The listing builds one solid part. Answer for the finished solid, in the listing's coordinates (mm). A direction names the side the tool comes from. Coordinates: 2 decimals unless noted, no trailing zeros. Loops run counter-clockwise (first coordinate to the right, second up) from the corner with the lowest first, then second, coordinate; pieces in that order, holes last. Notation, with made-up numbers: (-20.5, 42.5) -> (9.5, 42.5) arc R29 cw to (9.5, 80.5) -> close; hole circle Ø7 at (64.5, 76). An arc over 180 degrees is marked (long way). Answer in a Markdown table with one row per item.
```python
from build123d import *

# Parameters (mm, degrees)
F0_W     = 280
F0_H     = 180
F0_R     = 3.25
F0_R_2   = 2.5
F0_R_3   = 5
F0_R_4   = 26
F0_R_5   = 14
F1_DEPTH = 36
F2_DEPTH = 18
F3_DEPTH = 10
F4_D     = 5
F4_DEPTH = 10
F4_TIP   = 1.5021515476
F5_R     = 19
F5_R_2   = 14
F6_DEPTH = 12
F8_R     = 20
F9_DEPTH = 2


with BuildPart() as f1:
    # F0 (on Top) → F1 (new body)
    with BuildSketch(Plane.XY):
        Rectangle(F0_W, F0_H)
        with Locations((-125, -70)):
            Circle(F0_R, mode=Mode.SUBTRACT)
        with Locations((-71.2132034356, -21.2132034356)):
            Circle(F0_R_2, mode=Mode.SUBTRACT)
        with Locations((-28.7867965644, -21.2132034356)):
            Circle(F0_R_2, mode=Mode.SUBTRACT)
        with Locations((125, -70)):
            Circle(F0_R, mode=Mode.SUBTRACT)
        with Locations((125, -55)):
            Circle(F0_R_3, mode=Mode.SUBTRACT)
        with Locations((28.7867965644, -21.2132034356)):
            Circle(F0_R_2, mode=Mode.SUBTRACT)
        with Locations((71.2132034356, -21.2132034356)):
            Circle(F0_R_2, mode=Mode.SUBTRACT)
        with Locations((-71.2132034356, 21.2132034356)):
            Circle(F0_R_2, mode=Mode.SUBTRACT)
        with Locations((-50, 0)):
            Circle(F0_R_4, mode=Mode.SUBTRACT)
        with Locations((-28.7867965644, 21.2132034356)):
            Circle(F0_R_2, mode=Mode.SUBTRACT)
        with Locations((-125, 55)):
            Circle(F0_R_3, mode=Mode.SUBTRACT)
        with Locations((-125, 70)):
            Circle(F0_R, mode=Mode.SUBTRACT)
        with Locations((28.7867965644, 21.2132034356)):
            Circle(F0_R_2, mode=Mode.SUBTRACT)
        with Locations((50, 0)):
            Circle(F0_R_4, mode=Mode.SUBTRACT)
        with Locations((71.2132034356, 21.2132034356)):
            Circle(F0_R_2, mode=Mode.SUBTRACT)
        with Locations((125, 70)):
            Circle(F0_R, mode=Mode.SUBTRACT)
        with Locations((-50, 0)):
            Circle(F0_R_4)
        with Locations((-50, 0)):
            Circle(F0_R_5, mode=Mode.SUBTRACT)
        with Locations((50, 0)):
            Circle(F0_R_4)
        with Locations((50, 0)):
            Circle(F0_R_5, mode=Mode.SUBTRACT)
        with Locations((-125, 55)):
            Circle(F0_R_3)
        with Locations((125, -55)):
            Circle(F0_R_3)
        with Locations((-71.2132034356, 21.2132034356)):
            Circle(F0_R_2)
        with Locations((-71.2132034356, -21.2132034356)):
            Circle(F0_R_2)
        with Locations((-28.7867965644, -21.2132034356)):
            Circle(F0_R_2)
        with Locations((-28.7867965644, 21.2132034356)):
            Circle(F0_R_2)
        with Locations((28.7867965644, 21.2132034356)):
            Circle(F0_R_2)
        with Locations((28.7867965644, -21.2132034356)):
            Circle(F0_R_2)
        with Locations((71.2132034356, -21.2132034356)):
            Circle(F0_R_2)
        with Locations((71.2132034356, 21.2132034356)):
            Circle(F0_R_2)
    extrude(amount=-F1_DEPTH)

    # F0 (on Top) → F2 (cut)
    with BuildSketch(Plane.XY):
        with Locations((-50, 0)):
            Circle(F0_R_4)
        with Locations((-50, 0)):
            Circle(F0_R_5, mode=Mode.SUBTRACT)
        with Locations((50, 0)):
            Circle(F0_R_4)
        with Locations((50, 0)):
            Circle(F0_R_5, mode=Mode.SUBTRACT)
    extrude(amount=-F2_DEPTH, mode=Mode.SUBTRACT)

    # F0 (on Top) → F3 (cut)
    with BuildSketch(Plane.XY):
        with Locations((-125, 55)):
            Circle(F0_R_3)
        with Locations((125, -55)):
            Circle(F0_R_3)
    extrude(amount=-F3_DEPTH, mode=Mode.SUBTRACT)

    # F4
    with Locations(Plane.XY):
        with Locations((-71.2132034356, 21.2132034356), (-71.2132034356, -21.2132034356), (-28.7867965644, -21.2132034356), (-28.7867965644, 21.2132034356), (28.7867965644, 21.2132034356), (28.7867965644, -21.2132034356), (71.2132034356, -21.2132034356), (71.2132034356, 21.2132034356)):
            Hole(F4_D / 2, depth=F4_DEPTH)
            with Locations((0, 0, -(F4_DEPTH + F4_TIP / 2))):  # 118° drill point
                Cone(0, F4_D / 2, F4_TIP, mode=Mode.SUBTRACT)

    # F5 (on face) → F6 (cut)
    with BuildSketch(Plane(origin=(0, 0, -36), x_dir=(1, 0, 0), z_dir=(0, 0, -1))):
        with Locations((50, 0)):
            Circle(F5_R)
        with Locations((50, 0)):
            Circle(F5_R_2, mode=Mode.SUBTRACT)
        with Locations((-50, 0)):
            Circle(F5_R)
        with Locations((-50, 0)):
            Circle(F5_R_2, mode=Mode.SUBTRACT)
    extrude(amount=-F6_DEPTH, mode=Mode.SUBTRACT)

    # F8 (on offset) → F9 (cut)
    with BuildSketch(Plane.XY.offset(-32)):
        with Locations((-50, 0)):
            Circle(F8_R)
        with Locations((50, 0)):
            Circle(F8_R)
    extrude(amount=-F9_DEPTH, mode=Mode.SUBTRACT)


solid = f1.part
```
Item 1: A tool of negligible diameter and unlimited length cuts with its end or side. For faces 4 (the face through (-65.08, 11.56, -28.06)), 5 (the face through (129.77, -53.5, -4.93)), 6 (the face through (-32, -7, -34)), 7 (the face through (36.014, 0.616, -20.958)), from which of +Z, -Z, +X, -X, +Y, -Y can it reach the whole face along a straight path? Write none if from no direction.
Findings below:
| item | result |
|---|---|
| face 4 | -Z |
| face 5 | +Z |
| face 6 | none |
| face 7 | +Z, -Z |
Item 2: A cutting plane is placed at C-C, the plane x = -50. Determine the outline of the cut face in (y, z).
Findings below:
| item | result |
|---|---|
| outline | (-90, -36) -> (-19, -36) -> (-19, -34) -> (-20, -34) -> (-20, -32) -> (-19, -32) -> (-19, -24) -> (-14, -24) -> (-14, -18) -> (-26, -18) -> (-26, 0) -> (-90, 0) -> close; (14, -24) -> (19, -24) -> (19, -32) -> (20, -32) -> (20, -34) -> (19, -34) -> (19, -36) -> (90, -36) -> (90, 0) -> (26, 0) -> (26, -18) -> (14, -18) -> close |
Item 3: Determine the mould class of faces 1 (the face through (-2, 90, -18)), 2 (the face through (140, -1, -18)), 3 (the face through (68, -7, -34)) for opening direction X: +X half, -X half, draft (parallel to the pull), parting line (faces both ways), or undercut.
Findings below:
| item | result |
|---|---|
| face 1 | draft |
| face 2 | +X half |
| face 3 | undercut |
Item 4: A cutting plane is placed at A-A, the plane x = 125. Determine the outline of the cut face in (y, z).
Findings below:
| item | result |
|---|---|
| outline | (-90, -36) -> (-73.25, -36) -> (-73.25, 0) -> (-90, 0) -> close; (-66.75, -36) -> (66.75, -36) -> (66.75, 0) -> (-50, 0) -> (-50, -10) -> (-60, -10) -> (-60, 0) -> (-66.75, 0) -> close; (73.25, -36) -> (90, -36) -> (90, 0) -> (73.25, 0) -> close |
Item 5: A cutting plane is placed at B-B, the plane y = -70. Determine the outline of the cut face in (x, z).
Findings below:
| item | result |
|---|---|
| outline | (-140, -36) -> (-128.25, -36) -> (-128.25, 0) -> (-140, 0) -> close; (-121.75, -36) -> (121.75, -36) -> (121.75, 0) -> (-121.75, 0) -> close; (128.25, -36) -> (140, -36) -> (140, 0) -> (128.25, 0) -> close |
Item 6: A cutting plane is placed at D-D, the plane z = -7. Count the separate pieces of the cut face and the enclosed holes in it, plus the area to 3 significant figures.
Findings below:
| item | result |
|---|---|
| separate pieces | 1 |
| enclosed holes | 16 |
| area | 45,700 mm2 |
Item 7: Find the intervals of material crossed by probe 1 along X at (y, z) = (0, -30); probe 2 along Y at (x, z) = (125, -3); probe 3 along X at (y, z) = (-1, -3), in increasing order.
Findings below:
| item | result |
|---|---|
| probe 1 | x = -140 to -69, -31 to 31, 69 to 140 |
| probe 2 | y = -90 to -73.25, -66.75 to -60, -50 to 66.75, 73.25 to 90 |
| probe 3 | x = -140 to -75.98, -24.02 to 24.02, 75.98 to 140 |
Item 8: Flat-ended cylindrical pins translate along their axes: pin 1 Ø8 at (x, y) = (-125, 55) entering from +Z; pin 2 Ø20 at (x, y) = (49, -2.5) entering from -Z. Find the tip coordinate at first contact, or state that the pin passes through.
Findings below:
| item | result |
|---|---|
| pin 1 | stops at z = -10 |
| pin 2 | passes through |
